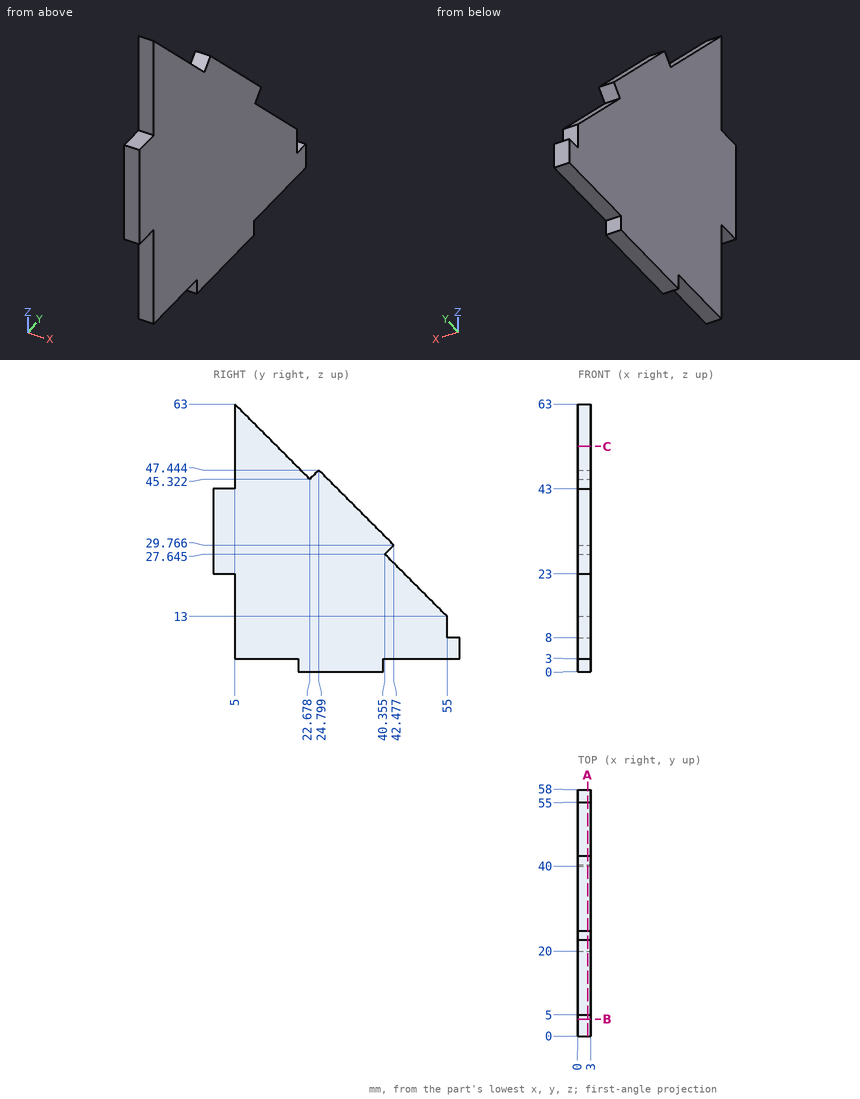
Verification items for this drawing (mm, ordinates from the low corner). Coordinates: 2 decimals unless noted, no trailing zeros. Loops run counter-clockwise (first coordinate to the right, second up) from the corner with the lowest first, then second, coordinate; pieces in that order, holes last.
Item 1: Thickness scan on line 1 (Y direction, x = 1.9, z = 4.5); line 2 (Y direction, x = 1.8, z = 46.5) (1 decimal); line 3 (Z direction, x = 0.8, y = 3). Record the ranges inside material, lowest first.
Item 2: Sectioned sample at A-A, the plane x = 2.3. Record the boundary of the cut face in (y, z) (1 decimal), then the cut area to 3 significant figures.
Item 3: Go/stop test with flat-tipped pins: pin 1 Ø1.5 at (x, z) = (1.5, 9.5) entering from +Y; pin 2 Ø0.9 at (x, y) = (2, 50) entering from -Z; pin 3 Ø1 at (x, y) = (1.5, 12) entering from +Z. Record where each tip stops, or that it passes through.
Item 4: Sectioned sample at C-C, the plane z = 53. Record the boundary of the cut face in (x, y), then the cut area to 3 significant figures.
Item 5: Sectioned sample at B-B, the plane y = 4. Record the boundary of the cut face in (x, z).
Check result:
1. line 1: y = 5 to 58
1. line 2: y = 5 to 21.5, 23.9 to 25.7
1. line 3: z = 23 to 43
2. outline: (0, 23) - (5, 23) - (5, 3) - (20, 3) - (20, 0) - (40, 0) - (40, 3) - (58, 3) - (58, 8) - (55, 8) - (55, 13) - (40.4, 27.6) - (42.5, 29.8) - (24.8, 47.4) - (22.7, 45.3) - (5, 63) - (5, 43) - (0, 43) - close
2. area: 2,000 mm2
3. pin 1: stops at y = 55
3. pin 2: stops at z = 3
3. pin 3: stops at z = 56.5
4. outline: (0, 5) - (3, 5) - (3, 15) - (0, 15) - close
4. area: 30.0 mm2
5. outline: (0, 23) - (3, 23) - (3, 43) - (0, 43) - close
